Can you work these out from the model? Positions are in its coordinate system, mm. A direction names the side the tool comes from. Coordinates: 2 decimals unless noted, no trailing zeros. Loops run counter-clockwise (first coordinate to the right, second up) from the corner with the lowest first, then second, coordinate; pieces in that order, holes last.
Autodesk Inventor part; units mm, degrees
ref_plane "YZ Plane" through (0, 0, 0) normal (1, 0, 0) x (0, 1, 0)
ref_plane "XZ Plane" through (0, 0, 0) normal (0, 1, 0) x (-1, 0, 0)
ref_plane "XY Plane" through (0, 0, 0) normal (0, 0, 1) x (1, 0, 0)
sketch "Sketch1" plane through (0, 0, 0) normal (0, 1, 0) x (-1, 0, 0)
  line L0 (-5, 26.5) -> (5, 26.5)
  line L1 (5, 26.5) -> (5, -26.5)
  line L2 (5, -26.5) -> (-5, -26.5)
  line L3 (-5, -26.5) -> (-5, 26.5)
  line L4 (5, -26.5) -> (5, -30.9444)
  line L5 (5, -30.9444) -> (-5, -26.5)
  line L6 (5, -30.9444) -> (5, 46.5)
  line L7 (5, 46.5) -> (-5, 26.5)
  line L8 (-5, -26.5) -> (0, -26.5)
  line L9 (-5, -21.5) -> (-5, -26.5)
  line L10 (5, 26.5) -> (0, 26.5)
  line L11 (5, 21.5) -> (5, 26.5)
  circle A0 centre (0, 21.5) radius 1.25
  circle A1 centre (0, -21.5) radius 1.25
  point P0 (0, 0)
  dimension "d0" = 10
  dimension "d1" = 53
  dimension "d2" = 4.4444
  dimension "d3" = 77.4444
  dimension "d8" = 2.5
  dimension "d9" = 2.5
extrude "Extrusion1" add sketch "Sketch1" along normal blind 50
sketch "Sketch2" plane through (5, 0, 26.5) normal (1, 0, 0) x (0, 0, -1)
  line L0 (53, 0) -> (0, 0)
  line L1 (0, 0) -> (0, 50)
  line L2 (0, 50) -> (53, 50)
  line L3 (53, 50) -> (53, 0)
  line L4 (26.5, 0) -> (26.5, 25)
  circle A0 centre (26.5, 25) radius 7.5
  circle A1 centre (26.5, 25) radius 5
  dimension "d12" = 25
  dimension "d13" = 15
  dimension "d16" = 10
extrude "Extrusion2" cut sketch "Sketch2" against normal blind 10 contours A1 | A0
extrude "Extrusion3" add sketch "Sketch2" against normal blind 2 contours A0
properties part number "bocnice_kratsi"
(1) I want a section at A-A on y = 25. Write out the boundary of the cut face in (x, z).
Check values:
outline: (-5, -30.94) - (5, -26.5) - (5, -5) - (3, -5) - (3, -7.5) - (-5, -7.5) - close; (-5, 7.5) - (3, 7.5) - (3, 5) - (5, 5) - (5, 26.5) - (-5, 46.5) - close; hole circle Ø2.5 at (0, -21.5); hole circle Ø2.5 at (0, 21.5)
(2) I'm going to push flat-ended pins straight in: pin 1 (1 mm diameter, centred on x = 3, z = 28, fed in from -Y); pin 2 (6 mm diameter, centred on y = 25, z = 0, fed in from +X); pin 3 (3 mm diameter, centred on x = -1, y = 40.5, fed in from +Z); pin 4 (6 mm diameter, centred on x = 2.5, y = 11, fed in from +Z). Where does each tip first touch, or does it pass through?
Check values:
pin 1: stops at y = 0
pin 2: passes through
pin 3: stops at z = 41.5
pin 4: stops at z = 37.5
(3) Which directions (+Z, -Z, +X, -X, +Y, -Y) give clear straight access to the entire face, cutting with the end or side of a thin tool? Please do faces 1 (the flat face through (-0.07, 24.65, 36.64)), 2 (the flat face through (3, 23, -5)).
Check values:
face 1: +Z, +X, +Y, -Y
face 2: -X
(4) I want a section at C-C on z = -21.5. Write out the boundary of the cut face in (x, y).
Check values:
outline: (-5, 0) - (-1.25, 0) - (-1.25, 50) - (-5, 50) - close; (1.25, 0) - (5, 0) - (5, 50) - (1.25, 50) - close
(5) I want a section at D-D on z = 0. Write out the boundary of the cut face in (x, y), then the cut area to 3 significant figures.
Check values:
outline: (-5, 0) - (5, 0) - (5, 20) - (3, 20) - (3, 17.5) - (-5, 17.5) - close; (-5, 32.5) - (3, 32.5) - (3, 30) - (5, 30) - (5, 50) - (-5, 50) - close
area: 360 mm2
(6) I want a section at B-B on x = 0. Write out the boundary of the cut face in (y, z).
Check values:
outline: (0, -28.72) - (50, -28.72) - (50, -22.75) - (0, -22.75) - close; (0, -20.25) - (50, -20.25) - (50, 20.25) - (0, 20.25) - close; (0, 22.75) - (50, 22.75) - (50, 36.5) - (0, 36.5) - close; hole circle Ø15 at (25, 0)
(7) If I drill on probe 1 along Z at (x, y) = (0.5, 46.5); probe 2 along Z at (x, y) = (0, 11.5); probe 3 along Y at (x, z) = (-2.75, 0), over which ranges is the centre line in solid material (lowest first)?
Check values:
probe 1: z = -28.5 to -22.65, -20.35 to 20.35, 22.65 to 35.5
probe 2: z = -28.72 to -22.75, -20.25 to 20.25, 22.75 to 36.5
probe 3: y = 0 to 17.5, 32.5 to 50
(8) If we mould it in two halves opening along Y, with no side actions, what happens to faces 3 (the flat face through (0, 50, 0)), 4 (the cylindrical face through (-0.944, 32.436, 0.976)), 5 (the cylindrical face through (0.27, 24.65, -20.28))? For each: released by +Y, released by -Y, zero draft, split by the parting line, or undercut.
Check values:
face 3: released by +Y
face 4: undercut
face 5: zero draft
